from build123d import *

# Parameters (mm, degrees)
SKETCH_1_W      = 65
SKETCH_1_H      = 65
SKETCH_1_R      = 11
EXTRUDE_1_DEPTH = 30
CHAMFER_1_SIZE  = 2


with BuildPart() as part:
    # Эскиз1 → Бобышка-Вытянуть1 (new body)
    with BuildSketch(Plane.XY):
        Rectangle(SKETCH_1_W, SKETCH_1_H)
        Circle(SKETCH_1_R, mode=Mode.SUBTRACT)
    extrude(amount=EXTRUDE_1_DEPTH)

    # Фаска1
    chamfer_1_edges = [part.edges().sort_by_distance(p)[0] for p in [
        (-11, 0, 0),
        (-11, 0, 30),
    ]]
    chamfer(chamfer_1_edges, length=CHAMFER_1_SIZE)


solid = part.part
Could you check a few things on this model? Use its own coordinates, in mm. Give positions to 0.01 mm unless a question says otherwise; leave off trailing zeros. Order: outer loops, then holes, each group sorted by start corner. A loop starts at its lowest first (then second) coordinate and runs counter-clockwise, first axis right, second up.
1. Suppose I cut it at C-C (z = 26.5). List the corners of the cut face in (x, y) for me.
2. I need wall thicknesses on L1, parallel to Y at x = 0, z = 19.25; L2, parallel to X at y = 9.5, z = 28.75; L3, parallel to Y at x = -5, z = 26.25. Which ranges of each line are inside material? Lowest first, please.
3. Suppose I cut it at A-A (x = 0). List the corners of the cut face in (y, z) for me, plus the area to 3 significant figures.
4. Will this pin go through, and if not, where does the flat tip stop? P1, Ø20, axis at x = 0, y = 0, coming from the -Z side.
5. We'd pull the mould along Y, two halves only. Please class faces 1 (the flat face through (0, -32.5, 15)), 2 (the conical face through (-8.829, -6.769, 28.125)), 3 (the flat face through (-15, 0, 0)), 4 (the cylindrical face through (-2.38, -10.74, 14.82)): pulls with the +Y half, pulls with the -Y half, needs draft (parallel to the pull), parting line crosses it, or undercut.
Solved:
1. outline: (-32.5, -32.5) - (32.5, -32.5) - (32.5, 32.5) - (-32.5, 32.5) - close; hole circle Ø22 at (0, 0)
2. L1: y = -32.5 to -11, 11 to 32.5
2. L2: x = -32.5 to -6.91, 6.91 to 32.5
2. L3: y = -32.5 to -9.8, 9.8 to 32.5
3. outline: (-32.5, 0) - (-13, 0) - (-11, 2) - (-11, 28) - (-13, 30) - (-32.5, 30) - close; (11, 2) - (13, 0) - (32.5, 0) - (32.5, 30) - (13, 30) - (11, 28) - close
3. area: 1,280 mm2
4. P1: passes through
5. face 1: pulls with the -Y half
5. face 2: undercut
5. face 3: needs draft
5. face 4: undercut
